from build123d import *

# Parameters (mm, degrees)
F0_W     = 75.02421
F0_H     = 100.512072
F1_DEPTH = 5.08
F2_R     = 7.62
F3_SIZE  = 1.27
F4_R     = 2.129316
F5_DEPTH = 0.254
F6_SIZE  = 1.27


with BuildPart() as f1:
    # F0 (on Front) → F1 (new body)
    with BuildSketch(Plane.XZ):
        Rectangle(F0_W, F0_H)
    extrude(amount=F1_DEPTH)

    # F2
    f2_edges = [f1.edges().sort_by_distance(p)[0] for p in [
        (-37.512105, -2.54, 50.256036),
        (-37.512105, -2.54, -50.256036),
        (37.512105, -2.54, 50.256036),
        (37.512105, -2.54, -50.256036),
    ]]
    fillet(f2_edges, radius=F2_R)

    # F3
    f3_edges = [f1.edges().sort_by_distance(p)[0] for p in [
        (0, -5.08, -50.256036),
        (-35.280259, -5.08, -48.02419),
        (35.280259, -5.08, -48.02419),
        (-37.512105, -5.08, 0),
        (37.512105, -5.08, 0),
        (-35.280259, -5.08, 48.02419),
        (35.280259, -5.08, 48.02419),
        (0, -5.08, 50.256036),
    ]]
    chamfer(f3_edges, length=F3_SIZE)

    # F4 (on face) → F5 (cut)
    with BuildSketch(Plane.XZ.offset(5.08)):
        with Locations((-20.219289, 45.626208)):
            Circle(F4_R)
    extrude(amount=-F5_DEPTH, mode=Mode.SUBTRACT)

    # F6
    f6_edges = [f1.edges().sort_by_distance(p)[0] for p in [
        (0, 0, -50.256036),
        (-35.280259, 0, -48.02419),
        (35.280259, 0, -48.02419),
        (-37.512105, 0, 0),
        (37.512105, 0, 0),
        (-35.280259, 0, 48.02419),
        (35.280259, 0, 48.02419),
        (0, 0, 50.256036),
    ]]
    chamfer(f6_edges, length=F6_SIZE)


solid = f1.part
Verification items for the finished model (mm, model axes). Coordinates: 2 decimals unless noted, no trailing zeros. Return JSON: item names as keys, results as strings.
1) Thickness scan on L1, parallel to X at y = -2.85, z = 44.5; L2, parallel to X at y = -0.5, z = 1.5; L3, parallel to Z at x = -21, y = -1. Record the ranges inside material, lowest first. Write a range as [from, to].
Answer list:
{"L1": "[-37.28, 37.28]", "L2": "[-36.74, 36.74]", "L3": "[-49.99, 49.99]"}
2) Release check for a two-part mould opening along Z. For faces 1 (the conical face through (-34.59, -0.36, 47.43)), 2 (the flat face through (-1, 0, 1)), 3 (the flat face through (-20, -4.826, 46)) record: +Z half, -Z half, draft (parallel to the pull), parting line (faces both ways), or undercut.
Answer list:
{"face 1": "+Z half", "face 2": "draft", "face 3": "undercut"}
3) Gauge pin test, flat end, axial feed: pin 1 (3.5 mm diameter, centred on x = -20.5, z = 45.5, fed in from -Y). Record the tip position at first contact, or that the pin passes through.
Answer list:
{"pin 1": "y = -4.83"}
